Source: CAD feature listing. Evaluate the final solid. Frame: model axes, mm. Give positions to 0.01 mm unless a question says otherwise; leave off trailing zeros. Write each loop counter-clockwise with the first axis right and the second up, starting at its lowest first coordinate (ties: lowest second). Pieces come first, ordered by that corner, then holes. Notation, with made-up numbers: (-12.5, -35) -> (18.5, -35) arc R7 ccw to (18.5, -30) -> close; hole circle Ø3 at (-28.5, -14). An arc over 180 degrees is marked (long way). Use one line per item in the form item = value. Start each with the question number.
(1) Material intervals for line 1 along Z through (x, y) = (-30, 4.25); line 2 along Y through (x, z) = (55, -31), sorted ascending. Write a range as from..to.
(2) Cut plane B-B, the plane z = 27. Output: boundary loops of the cut face in (x, y).
(3) First-contact query: P1, Ø4, axis at x = 33.5, z = -22, coming from the -Y side; P2, Ø1.5, axis at x = 58, z = -28, coming from the +Y side. Flat tips, straight axial feed; report the tip coordinate or a pass-through.
(4) Cut plane A-A, the plane x = -51. Output: boundary loops of the cut face in (y, z).
from build123d import *
from OCP.BRepFilletAPI import BRepFilletAPI_MakeChamfer

# Parameters (mm, degrees)
SKETCH1_W           = 160
SKETCH1_H           = 88
BOSS_EXTRUDE1_DEPTH = 0.6
SKETCH2_W           = 160
SKETCH2_H           = 1
BOSS_EXTRUDE2_DEPTH = 8.6
SKETCH3_R           = 1.25
BOSS_EXTRUDE3_DEPTH = 1.5
BOSS_EXTRUDE4_START = 1.5
SKETCH4_R           = 1.25
BOSS_EXTRUDE4_DEPTH = 1.5
CHAMFER1_SIZE       = 8
CHAMFER1_SIZE2      = 2.911761874
SKETCH5_W           = 140
SKETCH5_H           = 5
CUT_EXTRUDE1_DEPTH  = 1.5
FILLET1_R           = 2


with BuildPart() as part:
    # Sketch1 → Boss-Extrude1 (new body)
    with BuildSketch(Plane(origin=(0, 0, 0), x_dir=(1, 0, 0), z_dir=(0, 1, 0))):
        Rectangle(SKETCH1_W, SKETCH1_H)
    extrude(amount=BOSS_EXTRUDE1_DEPTH)

    # Sketch2 → Boss-Extrude2 (add)
    with BuildSketch(Plane(origin=(0, 0.6, 0), x_dir=(1, 0, 0), z_dir=(0, 1, 0))):
        with Locations((0, 43.5)):
            Rectangle(SKETCH2_W, SKETCH2_H)
        with Locations((0, -43.5)):
            Rectangle(SKETCH2_W, SKETCH2_H)
    extrude(amount=BOSS_EXTRUDE2_DEPTH)

    # Sketch3 → Boss-Extrude3 (add)
    with BuildSketch(Plane.XY.offset(-43)):
        with Locations(Location((-69, 4.6, 0), (0, 0, 180))):
            Circle(SKETCH3_R)
        with Locations(Location((69, 4.6, 0), (0, 0, 180))):
            Circle(SKETCH3_R)
    extrude(amount=BOSS_EXTRUDE3_DEPTH)

    # Sketch4 → Boss-Extrude4 (add)
    with BuildSketch(Plane(origin=(0, 0, 43), x_dir=(-1, 0, 0), z_dir=(0, 0, -1)).offset(BOSS_EXTRUDE4_START)):
        with Locations((-69, 4.6)):
            Circle(SKETCH4_R)
        with Locations((69, 4.6)):
            Circle(SKETCH4_R)
    extrude(amount=-BOSS_EXTRUDE4_DEPTH)

    # Chamfer1: one chamfer whose edges measure the first distance from different faces: ONE call of the kernel's chamfer builder (chamfer() names one face for all edges)
    chamfer1_edges_1 = [part.edges().sort_by_distance(p)[0] for p in [
        (-80, 9.2, -43.5),
        (-80, 9.2, 43.5),
    ]]
    chamfer1_side_1 = [part.faces().sort_by_distance(p)[0] for p in [
        (-80, 4.6, -43.115203978),
    ]]
    chamfer1_edges_2 = [part.edges().sort_by_distance(p)[0] for p in [
        (80, 9.2, -43.5),
        (80, 9.2, 43.5),
    ]]
    chamfer1_side_2 = [part.faces().sort_by_distance(p)[0] for p in [
        (80, 4.6, 43.115203978),
    ]]
    chamfer1 = BRepFilletAPI_MakeChamfer(part.part.solid().wrapped)
    for e in chamfer1_edges_1:
        chamfer1.Add(CHAMFER1_SIZE, CHAMFER1_SIZE2, e.wrapped, chamfer1_side_1[0].wrapped)  # the first distance lies on this face
    for e in chamfer1_edges_2:
        chamfer1.Add(CHAMFER1_SIZE, CHAMFER1_SIZE2, e.wrapped, chamfer1_side_2[0].wrapped)  # the first distance lies on this face
    add(Compound.cast(chamfer1.Shape()), mode=Mode.REPLACE)

    # Sketch5 → Cut-Extrude1 (cut)
    with BuildSketch(Plane(origin=(0, 0.6, 0), x_dir=(1, 0, 0), z_dir=(0, 1, 0))):
        Rectangle(SKETCH5_W, SKETCH5_H)
    extrude(amount=-CUT_EXTRUDE1_DEPTH, mode=Mode.SUBTRACT)

    # Fillet1
    fillet1_edges = [part.edges().sort_by_distance(p)[0] for p in [
        (70, 0.3, -2.5),
        (70, 0.3, 2.5),
        (-70, 0.3, 2.5),
        (-70, 0.3, -2.5),
    ]]
    fillet(fillet1_edges, radius=FILLET1_R)


solid = part.part
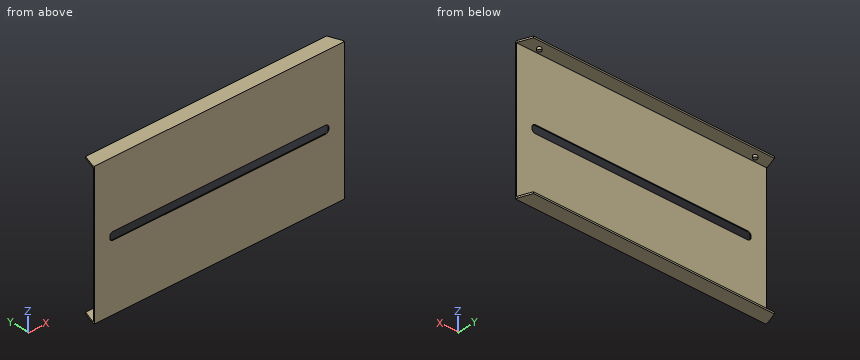
Geometry says:
q1.line_1 = -44..-43, 43..44
q1.line_2 = 0..0.6
q2.outline = (-80, 0) -> (80, 0) -> (80, 0.6) -> (-80, 0.6) -> close
q3.P1 = 0
q3.P2 = 0.6
q4.outline = (0, -44) -> (9.2, -44) -> (9.2, -43) -> (0.6, -43) -> (0.6, -2.5) -> (0, -2.5) -> close; (0, 2.5) -> (0.6, 2.5) -> (0.6, 43) -> (9.2, 43) -> (9.2, 44) -> (0, 44) -> close
